Part model, mm, in its own coordinate system. A direction names the side the tool comes from. Give positions to 0.01 mm unless a question says otherwise; leave off trailing zeros. Loops run counter-clockwise (first coordinate to the right, second up) from the corner with the lowest first, then second, coordinate; pieces in that order, holes last. Notation, with made-up numbers: (83.5, 11.5) -> (116.5, 11.5) arc R21 cw to (116.5, 45.5) -> close; hole circle Ø8 at (63, -15.75). An arc over 180 degrees is marked (long way). One line per question, with ' | ' between items.
Autodesk Inventor part; units mm, degrees
ref_plane "YZ Plane" through (0, 0, 0) normal (1, 0, 0) x (0, 1, 0)
ref_plane "XZ Plane" through (0, 0, 0) normal (0, 1, 0) x (-1, 0, 0)
ref_plane "XY Plane" through (0, 0, 0) normal (0, 0, 1) x (1, 0, 0)
sketch "Sketch1" plane through (0, 0, 0) normal (1, 0, 0) x (0, 1, 0)
  line L0 (0, 0) -> (25.4, 0)
  line L1 (25.4, 0) -> (25.4, 25.4)
  line L2 (25.4, 25.4) -> (0, 25.4)
  line L3 (0, 25.4) -> (0, 0)
  line L4 (1.651, 1.651) -> (23.749, 1.651)
  line L5 (23.749, 1.651) -> (23.749, 23.749)
  line L6 (23.749, 23.749) -> (1.651, 23.749)
  line L7 (1.651, 23.749) -> (1.651, 1.651)
  dimension "d0" = 25.4
  dimension "d2" = 25.4
  dimension "d3" = 1.651
  dimension "d4" = 1.651
  dimension "d5" = 1.651
  dimension "d6" = 1.651
extrude "Extrusion1" add sketch "Sketch1" along normal blind 914.4
sketch "Sketch3" plane through (0, 0, 0) normal (0, 0, -1) x (-1, 0, 0)
  line L0 (0, 25.4) -> (-914.4, 25.4)
  line L1 (-914.4, 0) -> (-914.4, 25.4)
  line L2 (0, 0) -> (-914.4, 0)
  point P0 (-889, 12.7)
  point P1 (-838.2, 12.7)
  dimension "d9" = 12.7
  dimension "d10" = 25.4
  dimension "d11" = 12.7
  dimension "d12" = 50.8
hole "Hole1" at (889, 12.7, 0) at (838.2, 12.7, 0) direction (0, 0, 1) diameter 6.35 end through all
sketch "Sketch4" plane through (0, 25.4, 25.4) normal (0, 1, 0) x (1, 0, 0)
  line L0 (0, 0) -> (914.4, 0)
  line L1 (914.4, 25.4) -> (914.4, 0)
  line L2 (0, 25.4) -> (914.4, 25.4)
  line L3 (736.6, 25.4) -> (736.6, 0)
  point P0 (711.2, 12.7)
  point P1 (762, 12.7)
  dimension "d21" = 50.8
  dimension "d23" = 12.7
  dimension "d24" = 12.7
  dimension "d25" = 177.8
  dimension "d26" = 25.4
hole "Hole2" at (711.2, 25.4, 12.7) at (762, 25.4, 12.7) direction (0, -1, 0) diameter 6.35 end through all
sketch "Sketch5" plane through (0, 0, 0) normal (0, 0, -1) x (-1, 0, 0)
  line L0 (0, 0) -> (0, 25.4)
  line L1 (0, 0) -> (-914.4, 0)
  point P0 (-314.7314, 12.7)
  point P1 (-22.6314, 12.7)
  dimension "d34" = 12.7
  dimension "d35" = 292.1
  dimension "d36" = 22.6314
hole "Hole3" at (314.7314, 12.7, 0) at (22.6314, 12.7, 0) direction (0, 0, 1) diameter 6.35 end through all
sketch "Sketch6" plane through (0, 0, 0) normal (0, -1, 0) x (1, 0, 0)
  line L0 (0, 0) -> (914.4, 0)
  line L1 (914.4, 25.4) -> (914.4, 0)
  line L2 (0, 25.4) -> (914.4, 25.4)
  point P0 (431.8, 12.7)
  point P1 (482.6, 12.7)
  dimension "d44" = 50.8
  dimension "d46" = 12.7
  dimension "d47" = 12.7
  dimension "d48" = 431.8
hole "Hole4" at (431.8, 0, 12.7) at (482.6, 0, 12.7) direction (0, 1, 0) diameter 6.35 end through all
sketch "Sketch7" plane through (0, 0, 25.4) normal (0, 0, 1) x (1, 0, 0)
  line L0 (914.4, 25.4) -> (914.4, 0)
  line L1 (0, 25.4) -> (914.4, 25.4)
  point P0 (457.2, 12.7)
  dimension "d56" = 12.7
  dimension "d57" = 457.2
hole "Hole5" at (457.2, 12.7, 25.4) direction (0, 0, -1) diameter 6.35 end through all
sketch "Sketch8" plane through (0, 0, 0) normal (0, -1, 0) x (1, 0, 0)
  line L0 (0, 25.4) -> (0, 0)
  point P0 (25.4, 12.7)
  point P1 (76.2, 12.7)
  dimension "d65" = 25.4
  dimension "d66" = 50.8
hole "Hole6" at (25.4, 0, 12.7) at (76.2, 0, 12.7) direction (0, 1, 0) diameter 6.35 end through all
properties part number "Bottom_Bar" material "Aluminum 6061"
1) Saw through at A-A (x = 559). Give the cut face in (y, z), and give its area (3 significant figures).
Found:
outline: (0, 0) -> (25.4, 0) -> (25.4, 25.4) -> (0, 25.4) -> close; hole (1.65, 1.65) -> (23.75, 1.65) -> (23.75, 23.75) -> (1.65, 23.75) -> close | area: 157 mm2
2) Pin check, flat tip, straight feed: P1, Ø5, axis at x = 22.63, y = 12.7, coming from the -Z side. Stop position of the tip, or through.
Found:
P1: through
3) Tool access for faces 5 (the flat face through (451, 0, 13)), 6 (the flat face through (451, 23.749, 13)): list every direction of +Z, -Z, +X, -X, +Y, -Y with a clear straight run to the whole face (end or side of a thin tool).
Found:
face 5: +Z, -Z, +X, -X, -Y | face 6: +X, -X
4) Pull direction Z, two halves, no side cores. Call faces 1 (the flat face through (451, 1.651, 13)), 2 (the flat face through (451, 13, 0)), 3 (the flat face through (451, 25.4, 13)), 4 (the flat face through (451, 13, 1.651)): pulls with the +Z half, pulls with the -Z half, needs draft (parallel to the pull), parting line crosses it, or undercut.
Found:
face 1: undercut | face 2: pulls with the -Z half | face 3: needs draft | face 4: undercut
5) Drill centre lines: line 1 (X direction, y = 12.7, z = 1.15) (3 decimals); line 2 (Z direction, x = 349, y = 21.5). Where is each one in solid material? Low to high.
Found:
line 1: 0 to 19.456, 25.806 to 311.556, 317.906 to 454.025, 460.375 to 835.025, 841.375 to 885.825, 892.175 to 914.4 | line 2: 0 to 1.65, 23.75 to 25.4
